```python
from build123d import *

# Parameters (mm, degrees)
SKETCH_1_W        = 50
SKETCH_1_H        = 2
EXTRUDE_1_DEPTH   = 10
EXTRUDE_1_2_DEPTH = 10
SKETCH_2_W        = 50
SKETCH_2_H        = 6.8
EXTRUDE_2_DEPTH   = 2
FILLET_1_R        = 2


with BuildPart() as part:
    # Sketch 1 → Extrude 1 (new body)
    with BuildSketch(Plane.XY):
        with Locations((25, 1)):
            Rectangle(SKETCH_1_W, SKETCH_1_H)
    extrude(amount=EXTRUDE_1_DEPTH)



with BuildPart() as body_2:
    # Sketch 1 → Extrude 1 2 (new body)
    with BuildSketch(Plane.XY):
        with Locations((25, -3.8)):
            Rectangle(SKETCH_1_W, SKETCH_1_H)
    extrude(amount=EXTRUDE_1_2_DEPTH)


with BuildPart() as part_1:
    add(part.part)

    add(body_2.part)  # Extrude 2 merges body 2
    # Sketch 2 → Extrude 2 (add)
    with BuildSketch(Plane(origin=(0, 0, 0), x_dir=(-1, 0, 0), z_dir=(0, 0, -1))):
        with Locations((-25, -1.4)):
            Rectangle(SKETCH_2_W, SKETCH_2_H)
    extrude(amount=EXTRUDE_2_DEPTH)

    # Fillet 1
    fillet_1_edges = [part_1.edges().sort_by_distance(p)[0] for p in [
        (25, -2.8, 10),
        (25, 0, 10),
    ]]
    fillet(fillet_1_edges, radius=FILLET_1_R - 0.0001)  # a hair under: the kernel refuses the full size


solid = part_1.part
```
Verification items for the finished model (mm, model axes). A direction names the side the tool comes from. Coordinates: 2 decimals unless noted, no trailing zeros. Write each loop counter-clockwise with the first axis right and the second up, starting at its lowest first coordinate (ties: lowest second). Pieces come first, ordered by that corner, then holes. Notation, with made-up numbers: M 82.5,-33 L 103.5,-33 A8 ccw 103.5,-20 Z; hole C 80.25,46.5 d1. An arc over 180 degrees is marked long. One line per item, written item: value.
Item 1: Section check A-A, the plane z = 1. Record the boundary of the cut face in (x, y).
Check sheet entries:
outline: M 0,-4.8 L 50,-4.8 L 50,-2.8 L 0,-2.8 Z; M 0,0 L 50,0 L 50,2 L 0,2 Z
Item 2: Scan lines: line 1 along Y through (x, z) = (27, 6.5); line 2 along Z through (x, y) = (48.5, -1); line 3 along Y through (x, z) = (27.5, 9). Record each from-to range of solid material in increasing order.
Check sheet entries:
line 1: y = -4.8 to -2.8, 0 to 2
line 2: z = -2 to 0
line 3: y = -4.8 to -3.07, 0.27 to 2
Item 3: Section check C-C, the plane y = -0.5. Record the boundary of the cut face in (x, z), plus the area to 3 significant figures.
Check sheet entries:
outline: M 0,-2 L 50,-2 L 50,0 L 0,0 Z
area: 100 mm^2
Item 4: Mould release check, pull along Y, two halves, no side actions. Record for faces 1 (the flat face through (50, -3, 4)), 2 (the flat face through (25, 0, 4)), 3 (the flat face through (25, 2, 4)): pulls with the +Y half, pulls with the -Y half, needs draft (parallel to the pull), parting line crosses it, or undercut.
Check sheet entries:
face 1: needs draft
face 2: undercut
face 3: pulls with the +Y half
Item 5: Access from +Z, -Z, +X, -X, +Y, -Y to the whole of each face (thin tool, end or side, straight path). Record for faces 4 (the flat face through (25, -4.8, 4)), 5 (the cylindrical face through (25.35, 0.57, 9.4)).
Check sheet entries:
face 4: +Z, -Z, +X, -X, -Y
face 5: +Z, +X, -X
